Part print with two shaded views. Sizes in mm from the minimum x, y, z corner. A direction names the side the tool comes from. Round coordinates to 2 decimals unless told otherwise and drop trailing zeros. Loops run counter-clockwise (first coordinate to the right, second up) from the corner with the lowest first, then second, coordinate; pieces in that order, holes last. Notation, with made-up numbers: M 52.25,-34 L 101.25,-34 A11 ccw 101.25,-27 Z; hole C -16.75,65.5 d4. An arc over 180 degrees is marked long. Use a Markdown table: item, result. Add a question column.
Item 1: Wall check: L1, parallel to Y at x = 23.5, z = 8.5; L2, parallel to X at y = 15, z = 6.25; L3, parallel to Y at x = 8.5, z = 4.5. Give the ranges that are in metal, low to high. Write a range as from..to.
Item 2: Tool access for the marked faces 1 and 2: list every direction of +Z, -Z, +X, -X, +Y, -Y with a clear straight run to the whole face (end or side of a thin tool).
Item 3: Saw through at A-A on z = 2.5. Write the cut outline in (x, y).
Item 4: Pin check, flat tips, straight feed: P1, Ø2.5, axis at y = 11, z = 5.5, coming from the +X side; P2, Ø5, axis at x = 22, z = 7.5, coming from the +Y side; P3, Ø3, axis at y = 6, z = 6, coming from the +X side. Stop position of each tip, or through.
Item 5: Saw through at B-B on x = 7. Write the cut outline in (y, z).
Item 6: Saw through at C-C on y = 10. Write the cut outline in (x, z), then the cut area to 3 significant figures.
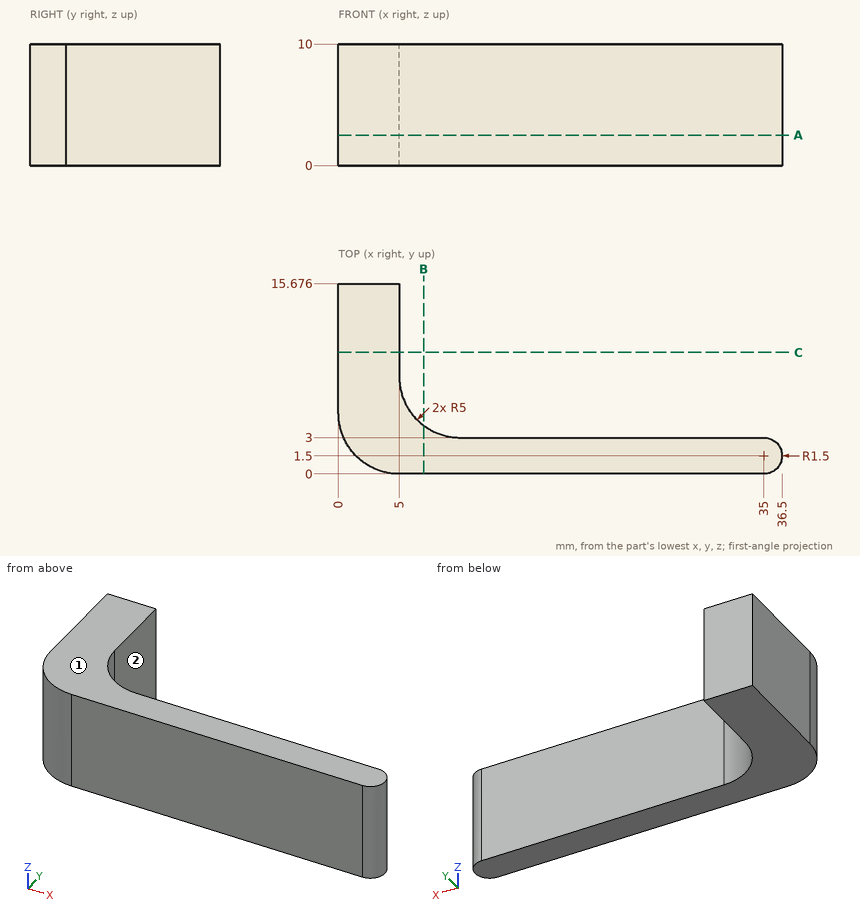
Entries:
| question | item | result |
|---|---|---|
| 1 | L1 | 0..3 |
| 1 | L2 | 0..5 |
| 1 | L3 | 0..3.23 |
| 2 | face 1 | +Z, +X, -X, +Y, -Y |
| 2 | face 2 | +Z, -Z, +X, +Y |
| 3 | outline | M 0,5 A5 ccw 5,0 L 35,0 A1.5 ccw 35,3 L 10,3 A5 cw 5,8 L 5,15.68 L 0,15.68 Z |
| 4 | P1 | x = 5 |
| 4 | P2 | y = 3 |
| 4 | P3 | x = 6.43 |
| 5 | outline | M 0,0 L 4,0 L 4,10 L 0,10 Z |
| 6 | outline | M 0,0 L 5,0 L 5,10 L 0,10 Z |
| 6 | area | 50.0 mm2 |
